from build123d import *

# Parameters (mm, degrees)
BOSS_EXTRUDE1_DEPTH = 15


with BuildPart() as part:
    # Sketch1 → Boss-Extrude1 (new, symmetric)
    with BuildSketch(Plane.XY):
        with BuildLine():
            Line((90, 65), (0, 65))
            ThreePointArc((0, 65), (-8.874119675, 62.093386622), (-14.309088021, 54.5))
            Line((-14.309088021, 54.5), (-28.618176043, 9))
            ThreePointArc((-28.618176043, 9), (-7.143700144, -29.137047693), (29.535645594, -5.25791207))
            ThreePointArc((29.535645594, -5.25791207), (50.100874494, 26.949083525), (87.406551135, 35.225900265))
            ThreePointArc((87.406551135, 35.225900265), (104.943418217, 48.698365648), (90, 65))
        make_face()
        with BuildLine():
            Line((50, 56), (90, 56))
            ThreePointArc((90, 56), (96, 50), (90, 44))
            Line((90, 44), (50, 44))
            ThreePointArc((50, 44), (44, 50), (50, 56))
        make_face(mode=Mode.SUBTRACT)
        with BuildLine():
            ThreePointArc((-14.956527547, 14.741176471), (0, -21), (14.956527547, 14.741176471))
            ThreePointArc((14.956527547, 14.741176471), (6.937432482, 29.759413292), (8.382229724, 46.723076923))
            ThreePointArc((8.382229724, 46.723076923), (0, 59), (-8.382229724, 46.723076923))
            ThreePointArc((-8.382229724, 46.723076923), (-6.937432482, 29.759413292), (-14.956527547, 14.741176471))
        make_face(mode=Mode.SUBTRACT)
    extrude(amount=BOSS_EXTRUDE1_DEPTH, both=True)


solid = part.part
Verification items for the finished model (mm, model axes). A direction names the side the tool comes from. Round coordinates to 2 decimals unless told otherwise and drop trailing zeros. Loops run counter-clockwise (first coordinate to the right, second up) from the corner with the lowest first, then second, coordinate; pieces in that order, holes last. Notation, with made-up numbers: (65.25, -26) - (88.25, -26) arc R26 ccw to (88.25, -11) - close; hole circle Ø4 at (30.25, -5). An arc over 180 degrees is marked (long way). Answer in a Markdown table with one row per item. Add a question column.
Q1. Tool access check on faces 5 (the face through (-21.363, 32.068, 0.21)), 6 (the face through (70, 44, 0)). Record the directions out of +Z, -Z, +X, -X, +Y, -Y that give a thin tool (end or side, any length) a straight path to the whole face; none if there is none.
Q2. Gauge pin test, flat ends, axial feed: pin 1 (9 mm diameter, centred on x = 67, z = -6.5, fed in from -Y); pin 2 (3 mm diameter, centred on y = 46.5, z = 0.5, fed in from +X); pin 3 (3 mm diameter, centred on y = 21, z = -12, fed in from +X). Record the tip position at first contact, or that the pin passes through.
Q3. Section check A-A on y = 25.5. Enter the section's corners in (x, z), plus the area to 3 significant figures.
Q4. Release check for a two-part mould opening along Y. For faces 1 (the face through (-0.69, -20.99, 0.21)), 2 (the face through (-9, 62, 0)), 3 (the face through (22, 29, -15)), 4 (the face through (49.65, 26.63, 0.21)) record: pulls with the +Y half, pulls with the -Y half, needs draft (parallel to the pull), parting line crosses it, or undercut.
Q5. Section check C-C on y = 0. Enter the section's corners in (x, z), plus the area to 3 significant figures.
Q6. Section check B-B on z = 1.25. Enter the section's corners in (x, y).
Q7. Material ranges on line 1 (X direction, y = 50, z = -3.5); line 2 (X direction, y = -6.5, z = 9.5); line 3 (X direction, y = 3, z = 11.25), recorded low to high.
Q8. Section check D-D on x = 23.5. Enter the section's corners in (y, z).
Found:
| question | item | result |
|---|---|---|
| 1 | face 5 | +Z, -Z, -X, +Y |
| 1 | face 6 | +Z, -Z |
| 2 | pin 1 | stops at y = 33.26 |
| 2 | pin 2 | stops at x = 104.87 |
| 2 | pin 3 | stops at x = 44.61 |
| 3 | outline | (-23.43, -15) - (-8.15, -15) - (-8.15, 15) - (-23.43, 15) - close; (8.15, -15) - (48.13, -15) - (48.13, 15) - (8.15, 15) - close |
| 3 | area | 1,660 mm² |
| 4 | face 1 | undercut |
| 4 | face 2 | pulls with the +Y half |
| 4 | face 3 | needs draft |
| 4 | face 4 | pulls with the -Y half |
| 5 | outline | (-30, -15) - (-21, -15) - (-21, 15) - (-30, 15) - close; (21, -15) - (30.77, -15) - (30.77, 15) - (21, 15) - close |
| 5 | area | 563 mm² |
| 6 | outline | (-28.62, 9) arc R30 ccw (long way) to (29.54, -5.26) arc R50 cw to (87.41, 35.23) arc R15 ccw (long way) to (90, 65) - (0, 65) arc R15 ccw to (-14.31, 54.5) - close; hole (-14.96, 14.74) arc R21 ccw (long way) to (14.96, 14.74) arc R30 cw to (8.38, 46.72) arc R9 ccw (long way) to (-8.38, 46.72) arc R30 cw to start; hole (50, 44) - (90, 44) arc R6 ccw to (90, 56) - (50, 56) arc R6 ccw to start |
| 7 | line 1 | x = -15.72 to -9, 9 to 44, 96 to 105 |
| 7 | line 2 | x = -29.29 to -19.97, 19.97 to 29.29 |
| 7 | line 3 | x = -29.85 to -20.78, 20.78 to 31.75 |
| 8 | outline | (-18.65, -15) - (65, -15) - (65, 15) - (-18.65, 15) - close |
